Could you check a few things on this drawing? It's one solid part, dimensions in mm from its lowest x, y, z. Round coordinates to 2 decimals unless told otherwise and drop trailing zeros. Write each loop counter-clockwise with the first axis right and the second up, starting at its lowest first coordinate (ties: lowest second). Pieces come first, ordered by that corner, then holes. Notation, with made-up numbers: (-39, 79.5) -> (-10, 79.5) arc R21 cw to (-10, 90.5) -> close; hole circle Ø6 at (24.25, 65.5). An arc over 180 degrees is marked (long way). Put each result on its own line as item: value. Start each with the question number.
1) We'd pull the mould along X, two halves only. Please class the marked faces 1, 2 and 3: released by +X, released by -X, zero draft, split by the parting line, or undercut.
2) Will these pins go through, and if not, where does the flat tip stop? P1, Ø11, axis at y = 92, z = 60, coming from the -X side; P2, Ø3, axis at x = 87.5, y = 72.5, coming from the -Z side; P3, Ø2, axis at y = 45, z = 34, coming from the +X side; P4, Ø10, axis at x = 79.5, z = 17, coming from the +Y side.
3) If I drill on line 1 along Y through (x, z) = (42, 75); line 2 along Z through (x, y) = (33, 93); line 3 along Z through (x, y) = (9, 62), over which ranges is the centre line in solid material (lowest first)? Write a range as [from, to].
4) I want a section at B-B, the plane x = 68.5. List the corners of the cut face in (y, z) for me.
5) I want a section at A-A, the plane y = 9. List the corners of the cut face in (x, z) for me, then the cut area to 3 significant figures.
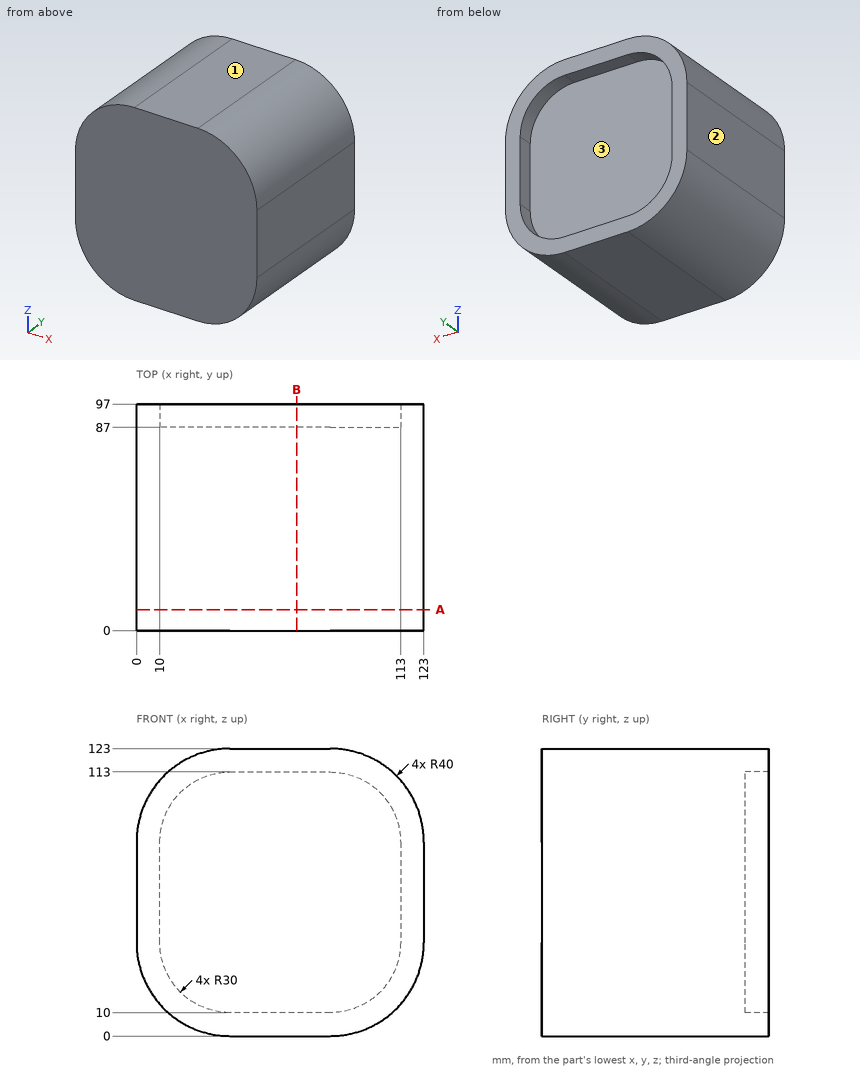
Findings:
1. face 1: zero draft
1. face 2: released by -X
1. face 3: undercut
2. P1: stops at x = 0
2. P2: stops at z = 0.11
2. P3: stops at x = 122.69
2. P4: stops at y = 87
3. line 1: y = [0, 87]
3. line 2: z = [0.62, 10.83], [112.17, 122.38]
3. line 3: z = [14.72, 108.28]
4. outline: (0, 0) -> (97, 0) -> (97, 10) -> (87, 10) -> (87, 113) -> (97, 113) -> (97, 123) -> (0, 123) -> close
5. outline: (0, 40) arc R40 ccw to (40, 0) -> (83, 0) arc R40 ccw to (123, 40) -> (123, 83) arc R40 ccw to (83, 123) -> (40, 123) arc R40 ccw to (0, 83) -> close
5. area: 13,800 mm2
